Source: CAD feature listing. Evaluate the final solid. Frame: model axes, mm. Face numbers are marked on the shaded views. Give positions to 0.01 mm unless a question says otherwise; leave off trailing zeros. Write each loop counter-clockwise with the first axis right and the second up, starting at its lowest first coordinate (ties: lowest second). Pieces come first, ordered by that corner, then holes. Notation, with made-up numbers: M 89.25,12 L 134.25,12 A19 ccw 134.25,23 Z; hole C -17.5,41 d11. An arc over 180 degrees is marked long. Return JSON: item names as keys, results as strings.
```python
from build123d import *

# Parameters (mm, degrees)
F0_R     = 25.4
F1_DEPTH = 2.54
F2_W     = 2.54
F2_H     = 2.54
F3_DEPTH = 25.4
F4_W     = 2.54
F4_H     = 2.54
F5_DEPTH = 25.4
F7_W     = 0.635
F7_H     = 2.54
F8_DEPTH = 25.4


with BuildPart() as f1:
    # F0 (on Top) → F1 (new body)
    with BuildSketch(Plane.XY):
        Circle(F0_R)
    extrude(amount=F1_DEPTH)

    # F2 (on face) → F3 (join)
    with BuildSketch(Plane(origin=(0, 0, 0), x_dir=(1, 0, 0), z_dir=(0, 0, -1))):
        with Locations((12.7, -12.7)):
            Rectangle(F2_W, F2_H)
        with Locations((-12.7, -12.7)):
            Rectangle(F2_W, F2_H)
        with Locations((-12.7, 12.7)):
            Rectangle(F2_W, F2_H)
        with Locations((12.7, 12.7)):
            Rectangle(F2_W, F2_H)
    extrude(amount=F3_DEPTH)

    # F4 (on face) → F5 (join)
    with BuildSketch(Plane(origin=(0, -11.43, 0), x_dir=(-1, 0, 0), z_dir=(0, 1, 0))):
        with Locations((12.7, -1.27)):
            Rectangle(F4_W, F4_H)
    extrude(amount=F5_DEPTH)

    # F6: F1 across plane


with BuildPart() as f1_1:
    add(f1.part)
    add(f1.part.mirror(Plane.YZ))

    # F7 (on face) → F8 (join)
    with BuildSketch(Plane.YZ.offset(-11.43)):
        with Locations((-1.0795, -1.27)):
            Rectangle(F7_W, F7_H)
    extrude(amount=F8_DEPTH)

    # F9: F1 across plane


with BuildPart() as f1_2:
    add(f1_1.part)
    add(f1_1.part.mirror(Plane.XZ))


solid = f1_2.part
```
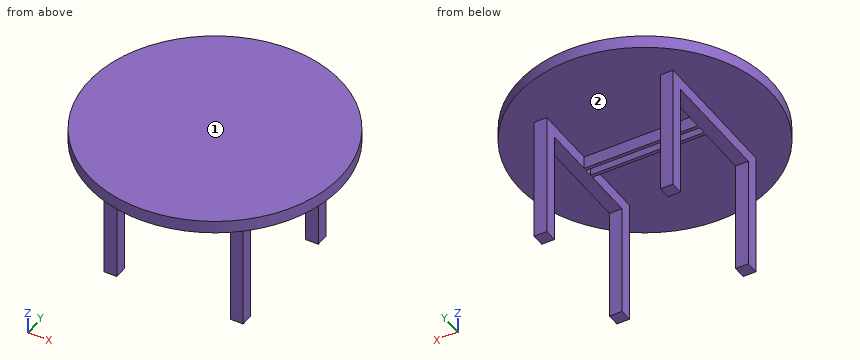
1) Contact query for flat-ended pins moving along their axis: pin 1 Ø0.8 at (x, z) = (2, -1.5) entering from -Y; pin 2 Ø0.8 at (x, z) = (-12.5, -7.5) entering from +Y; pin 3 Ø10 at (y, z) = (2.5, -12) entering from -X; pin 4 Ø2 at (x, z) = (12.5, -14) entering from -Y. Output: stop coordinate, or through.
Numbers:
{"pin 1": "stops at y = -1.4", "pin 2": "stops at y = 13.97", "pin 3": "passes through", "pin 4": "stops at y = -13.97"}
2) Cut plane B-B, the plane y = 0. Return the cut outline in (x, z).
Numbers:
{"outline": "M -25.4,0 L -13.97,0 L -13.97,-2.54 L -11.43,-2.54 L -11.43,0 L 11.43,0 L 11.43,-2.54 L 13.97,-2.54 L 13.97,0 L 25.4,0 L 25.4,2.54 L -25.4,2.54 Z"}
3) Line query: line 1 (Z direction, x = -15.5, y = 16); line 2 (Z direction, x = 13.5, y = 0); line 3 (Y direction, x = 17, z = 0.75). Output: solid intervals per line, ascending. Write a range as [from, to].
Numbers:
{"line 1": "z = [0, 2.54]", "line 2": "z = [-2.54, 2.54]", "line 3": "y = [-18.87, 18.87]"}
4) Draft query along X for the marked faces 1 and 2. Return one class per face: released by +X, released by -X, zero draft, split by the parting line, or undercut.
Numbers:
{"face 1": "zero draft", "face 2": "undercut"}
5) Cut plane C-C, the plane x = 0. Return the cut outline in (y, z), then the cut area to 3 significant figures.
Numbers:
{"outline": "M -25.4,0 L -1.4,0 L -1.4,-2.54 L -0.76,-2.54 L -0.76,0 L 0.76,0 L 0.76,-2.54 L 1.4,-2.54 L 1.4,0 L 25.4,0 L 25.4,2.54 L -25.4,2.54 Z", "area": "132 mm²"}
6) Cut plane A-A, the plane z = -16.5. Return the cut outline in (x, y).
Numbers:
{"outline": "M -13.97,-13.97 L -11.43,-13.97 L -11.43,-11.43 L -13.97,-11.43 Z; M -13.97,11.43 L -11.43,11.43 L -11.43,13.97 L -13.97,13.97 Z; M 11.43,-13.97 L 13.97,-13.97 L 13.97,-11.43 L 11.43,-11.43 Z; M 11.43,11.43 L 13.97,11.43 L 13.97,13.97 L 11.43,13.97 Z"}
7) Cut plane D-D, the plane z = -1. Return the cut outline in (x, y).
Numbers:
{"outline": "M -13.97,-13.97 L -11.43,-13.97 L -11.43,-1.4 L 11.43,-1.4 L 11.43,-13.97 L 13.97,-13.97 L 13.97,13.97 L 11.43,13.97 L 11.43,1.4 L -11.43,1.4 L -11.43,13.97 L -13.97,13.97 Z; hole M -11.43,-0.76 L 11.43,-0.76 L 11.43,0.76 L -11.43,0.76 Z"}
